The model under review builds one solid part; all positions refer to its coordinate system, in mm. A direction names the side the tool comes from. Coordinates: 2 decimals unless noted, no trailing zeros. Answer as a JSON object with one key per item and string values.
```python
from build123d import *

# Parameters (mm, degrees)
F0_W            = 98.3085063696
F0_H            = 59.0165173113
F0_W_2          = 92.3085063696
F0_H_2          = 53.0165173113
F1_DEPTH        = 8
F2_DEPTH        = 15
F3_R            = 5
F3_R_2          = 4
F4_DEPTH        = 6
F5_R            = 2.54
F6_R            = 3
F7_R            = 2.99999
F10_D           = 2.794
F10_CSINK_D     = 5.7404
F10_CSINK_ANGLE = 82


# Not quite as in the source:
# - a fillet or chamfer that OpenCascade refuses, or shapes differently, is made with other operations: its cross-section is extruded or revolved along the edge and cut away or added
# - a fillet or chamfer is up to 0.001 mm smaller than in the source, because OpenCascade refuses the exact size


with BuildPart() as f1:
    # F0 (on Front) → F1 (new body)
    with BuildSketch(Plane.XZ):
        Rectangle(F0_W, F0_H)
        Rectangle(F0_W_2, F0_H_2, mode=Mode.SUBTRACT)
        Rectangle(F0_W_2, F0_H_2)
    extrude(amount=F1_DEPTH)

    # F0 (on Front) → F2 (join)
    with BuildSketch(Plane.XZ):
        Rectangle(F0_W, F0_H)
        Rectangle(F0_W_2, F0_H_2, mode=Mode.SUBTRACT)
    extrude(amount=F2_DEPTH)

    # F3 (on face) → F4 (join)
    with BuildSketch(Plane.XZ.offset(8)):
        with Locations((-24.5116613805, 0)):
            Circle(F3_R)
        with Locations((-24.5116613805, 0)):
            Circle(F3_R_2, mode=Mode.SUBTRACT)
        with Locations((24.5116613805, 0)):
            Circle(F3_R)
        with Locations((24.5116613805, 0)):
            Circle(F3_R_2, mode=Mode.SUBTRACT)
    extrude(amount=F4_DEPTH)

    # F5
    f5_edges = [f1.edges().sort_by_distance(p)[0] for p in [
        (-29.511661, -8, 0),
        (19.511661, -8, 0),
        (0, -8, -26.508259),
        (46.154253, -8, 0),
        (-46.154253, -8, 0),
        (0, -8, 26.508259),
    ]]
    fillet(f5_edges, radius=F5_R)

    # F6
    f6_edges = [f1.edges().sort_by_distance(p)[0] for p in [
        (0, 0, 29.508259),
        (49.154253, 0, 0),
        (0, 0, -29.508259),
        (-49.154253, 0, 0),
    ]]
    fillet(f6_edges, radius=F6_R)

    # F7 (radius 3 in the source; OpenCascade refuses exactly that, so slightly less here)
    f7_edges = [f1.edges().sort_by_distance(p)[0] for p in [
        (0, -15, -29.508259),
        (49.154253, -15, 0),
        (-49.154253, -15, 0),
        (0, -15, 29.508259),
    ]]
    fillet(f7_edges, radius=F7_R)

    # F8: fillet of radius 2 on 2 edges, made by hand

    # F8_s1 → F8_t2 (revolve, cut)
    with BuildSketch(Plane.XY):
        with BuildLine():
            ThreePointArc((29.5120613805, -12.2673917434), (29.2440686279, -13.2678330874), (28.5118614771, -14.0003463544))
            Line((28.5118614771, -14.0003463544), (28.6119780552, -14.1736418155))
            ThreePointArc((28.6119780552, -14.1736418155), (29.0117614288, -14.2001365685), (29.5116613805, -14.2001365685))
            Line((29.5116613805, -14.2001365685), (29.7117979491, -14))
            ThreePointArc((29.7117979491, -14), (29.7117979491, -13.1336958717), (29.7121979491, -12.2673917434))
            Line((29.7121979491, -12.2673917434), (29.5120613805, -12.2673917434))
        make_face()
    revolve(axis=Axis((24.5116613805, -14, 0), (0, -1, 0)), mode=Mode.SUBTRACT)

    # F8_s3 → F8_t4 (revolve, cut)
    with BuildSketch(Plane.XY):
        with BuildLine():
            ThreePointArc((-19.5112613805, -12.2673917434), (-19.7792541332, -13.2678330874), (-20.511461284, -14.0003463544))
            Line((-20.511461284, -14.0003463544), (-20.4113447058, -14.1736418155))
            ThreePointArc((-20.4113447058, -14.1736418155), (-20.0115613323, -14.2001365685), (-19.5116613805, -14.2001365685))
            Line((-19.5116613805, -14.2001365685), (-19.311524812, -14))
            ThreePointArc((-19.311524812, -14), (-19.311524812, -13.1336958717), (-19.311124812, -12.2673917434))
            Line((-19.311124812, -12.2673917434), (-19.5112613805, -12.2673917434))
        make_face()
    revolve(axis=Axis((-24.5116613805, -14, 0), (0, -1, 0)), mode=Mode.SUBTRACT)

    # F10 (through all)
    with Locations(Plane.XZ.offset(8)):
        with Locations((37.2699052095, 16.8491732329), (37.2699052095, -16.8491732329), (0.4332323442, -16.7640619911), (0.4332323442, 16.9342844747), (-37.2699052095, 16.8491732329), (-37.2699052095, -16.8491732329)):
            CounterSinkHole(F10_D / 2, F10_CSINK_D / 2, counter_sink_angle=F10_CSINK_ANGLE)


solid = f1.part
```
(1) Wall thickness on line 1 along X through (y, z) = (-11.5, 9.5); line 2 along Z through (x, y) = (-26, -11); line 3 along Z through (x, y) = (20, -12.25): over which ranges is each line inside the solid? List them lowest first. Write a range as from..to.
Results list:
{"line 1": "-49.15..-46.15, 46.15..49.15", "line 2": "-29.51..-26.51, -4.77..-3.71, 3.71..4.77, 26.51..29.51", "line 3": "-29.5..-26.51, -2.16..2.16, 26.51..29.5"}
(2) Draft analysis for pull direction X (two halves, no side actions). For faces 3 (the face through (49.154, -7, 0)), 4 (the face through (38.666, -3.109, 16.911)), 5 (the face through (-48.299, -14.098, 0.413)), state which applies: released by +X, released by -X, zero draft, split by the parting line, or undercut.
Results list:
{"face 3": "released by +X", "face 4": "undercut", "face 5": "released by -X"}
(3) For pin 1 Ø1.7 at (x, z) = (0.43, -16.76) entering from +Y; pin 2 Ø4 at (x, z) = (-23.5, 1) entering from -Y; pin 3 Ø14.5 at (x, z) = (-15.5, -9) entering from -Y; pin 4 Ø6.5 at (x, z) = (26, 0) entering from -Y, all flat-tipped, find the tip position at first contact; note any pin that passes through.
Results list:
{"pin 1": "through", "pin 2": "y = -8", "pin 3": "y = -9.05", "pin 4": "y = -14"}
(4) For faces 1 (the face through (-1, -8, 0)), 2 (the face through (-49.154, -7, 0)), list the 3-axis set-ups (+Z, -Z, +X, -X, +Y, -Y) from which the entire face can be reached by the end or side of a thin tool; tool diameter is ignored.
Results list:
{"face 1": "-Y", "face 2": "+Z, -Z, -X, +Y, -Y"}
